Check sheet for the drawn part. Datum: minimum x, y, z corner. Units: mm. A direction names the side the tool comes from. Coordinates: 2 decimals unless noted, no trailing zeros. Order: outer loops, then holes, each group sorted by start corner. A loop starts at its lowest first (then second) coordinate and runs counter-clockwise, first axis right, second up. Notation, with made-up numbers: M -8.75,-6 L 15.25,-6 A31 cw 15.25,22 Z; hole C 20,4 d6. An arc over 180 degrees is marked long. Return JSON: item names as keys, results as strings. Group by question number.
Q1. Section check B-B, the plane x = 66.5. Enter the section's corners in (y, z) (1 decimal).
Q2. Thickness scan on probe 1 along X at (y, z) = (27.5, 45.5) (1 decimal); probe 2 along Z at (x, y) = (8.5, 44); probe 3 along Y at (x, z) = (8, 45) (1 decimal). Record the ranges inside material, lowest first.
Q3. Access from +Z, -Z, +X, -X, +Y, -Y to the whole of each face (thin tool, end or side, straight path). Record for the marked faces 1, 2 and 3.
Q4. Section check A-A, the plane x = 27. Enter the section's corners in (y, z), then the cut area to 3 significant figures.
Q5. Mould release check, pull along X, two halves, no side actions. Record for the marked faces 4, 5 and 6: pulls with the +X half, pulls with the -X half, needs draft (parallel to the pull), parting line crosses it, or undercut.
Q6. Go/stop test with flat-tipped pins: pin 1 Ø1.5 at (x, y) = (52.5, 45) entering from -Z; pin 2 Ø1.5 at (x, z) = (70, 27) entering from -Y; pin 3 Ø2 at (y, z) = (12, 52.5) entering from -X. Record where each tip stops, or that it passes through.
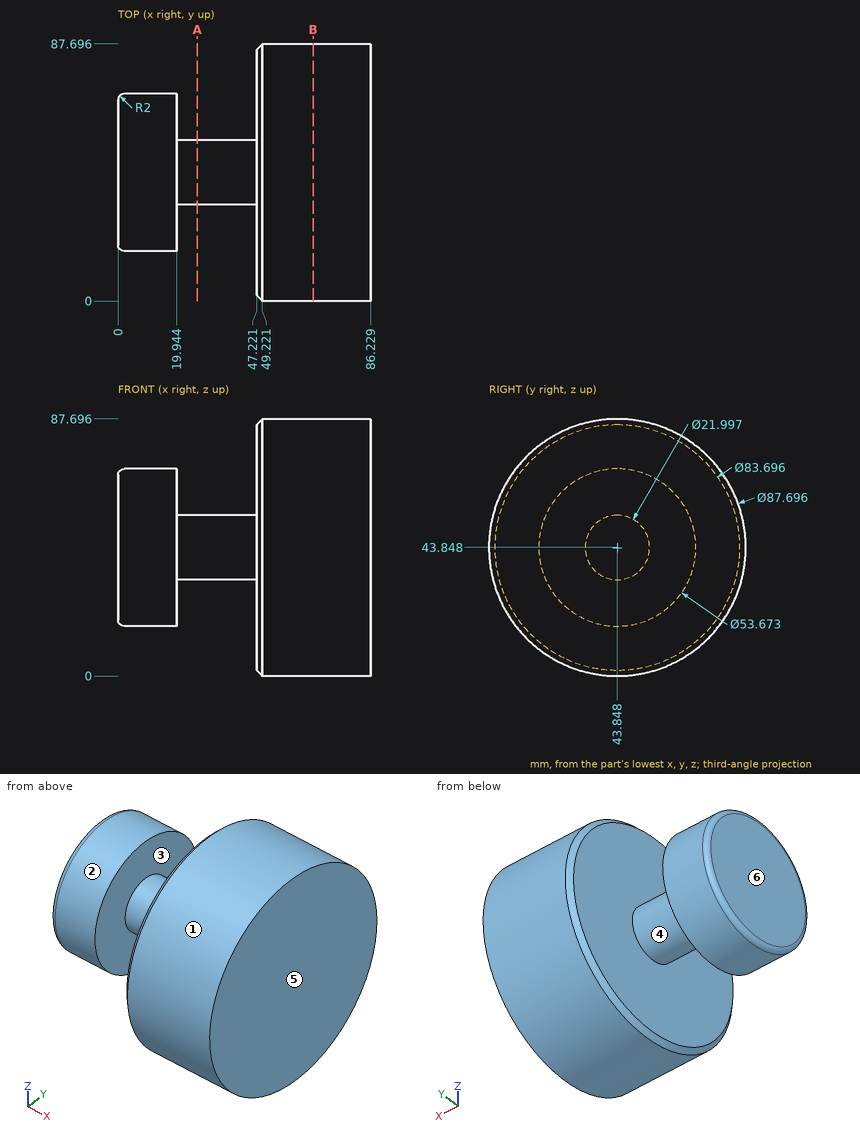
Numbers:
{
 "1": {"outline": "C 43.8,43.8 d87.7"},
 "2": {"probe 1": "x = 0 to 19.9, 47.2 to 86.2", "probe 2": "z = 17.01 to 70.68", "probe 3": "y = 17 to 70.7"},
 "3": {"face 1": "+X, -X", "face 2": "-X", "face 3": "none"},
 "4": {"outline": "C 43.85,43.85 d22", "area": "380 mm2"},
 "5": {"face 4": "undercut", "face 5": "pulls with the +X half", "face 6": "pulls with the -X half"},
 "6": {"pin 1": "stops at z = 0", "pin 2": "stops at y = 3.06", "pin 3": "stops at x = 47.22"}
}
